from build123d import *

# Parameters (mm, degrees)
F0_W     = 36
F0_H     = 36
F1_DEPTH = 36
F2_W     = 21
F2_H     = 21
F3_DEPTH = 60
F4_R     = 2.5
F5_DEPTH = 25
F6_R     = 2.5
F7_DEPTH = 20
F8_R     = 4.25
F9_DEPTH = 5.5


with BuildPart() as f1:
    # F0 (on Front) → F1 (new body)
    with BuildSketch(Plane.XZ):
        with Locations((18, 18)):
            Rectangle(F0_W, F0_H)
    extrude(amount=F1_DEPTH)

    # F2 (on face) → F3 (cut)
    with BuildSketch(Plane.YZ.offset(36)):
        with Locations((-18, 18)):
            Rectangle(F2_W, F2_H)
    extrude(amount=-F3_DEPTH, mode=Mode.SUBTRACT)

    # F4 (on face) → F5 (cut)
    with BuildSketch(Plane.XY.offset(36)):
        with Locations((18, -18)):
            Circle(F4_R)
    extrude(amount=-F5_DEPTH, mode=Mode.SUBTRACT)

    # F6 (on face) → F7 (cut)
    with BuildSketch(Plane.XZ.offset(36)):
        with Locations((18, 18)):
            Circle(F6_R)
    extrude(amount=-F7_DEPTH, mode=Mode.SUBTRACT)

    # F8 (on face) → F9 (cut)
    with BuildSketch(Plane.XZ.offset(36)):
        with Locations((18, 18)):
            Circle(F8_R)
    extrude(amount=-F9_DEPTH, mode=Mode.SUBTRACT)


solid = f1.part
Can you work these out from the model? Positions are in its coordinate system, mm. A direction names the side the tool comes from. Give positions to 0.01 mm unless a question says otherwise; leave off trailing zeros. Loops run counter-clockwise (first coordinate to the right, second up) from the corner with the lowest first, then second, coordinate; pieces in that order, holes last. Notation, with made-up numbers: (-14.75, -15.5) -> (12.25, -15.5) arc R21 ccw to (12.25, -8.5) -> close; hole circle Ø11 at (28, 62.25). An arc over 180 degrees is marked (long way). Use one line per item in the form item = value.
1) If we section it at B-B (y = -23): Please give me the cut outline in (x, z), plus the area to 3 significant figures.
Answers:
outline = (0, 0) -> (36, 0) -> (36, 7.5) -> (0, 7.5) -> close; (0, 28.5) -> (36, 28.5) -> (36, 36) -> (0, 36) -> close
area = 540 mm²
2) I need wall thicknesses on line 1 along Z through (x, y) = (18, -29); line 2 along Z through (x, y) = (18, -11.5); line 3 along Y through (x, z) = (18, 32). Which ranges of each line are inside material? Lowest first, please.
Answers:
line_1 = 0 to 15.5, 20.5 to 36
line_2 = 0 to 7.5, 28.5 to 36
line_3 = -36 to -20.5, -15.5 to 0
3) If we section it at C-C (x = 18): Please give me the cut outline in (y, z), plus the area to 3 significant figures.
Answers:
outline = (-36, 0) -> (0, 0) -> (0, 36) -> (-15.5, 36) -> (-15.5, 28.5) -> (-7.5, 28.5) -> (-7.5, 7.5) -> (-28.5, 7.5) -> (-28.5, 15.5) -> (-30.5, 15.5) -> (-30.5, 13.75) -> (-36, 13.75) -> close; (-36, 22.25) -> (-30.5, 22.25) -> (-30.5, 20.5) -> (-28.5, 20.5) -> (-28.5, 28.5) -> (-20.5, 28.5) -> (-20.5, 36) -> (-36, 36) -> close
area = 761 mm²
4) For faces 1 (the face through (15.5, -17.9, 32.3)), 2 (the face through (14, -28.5, 18)), 3 (the face through (16.16, -29.51, 19.69)), which set-ups out of +Z, -Z, +X, -X, +Y, -Y let a thin tool reach every point of the face, with its end or its side?
Answers:
face_1 = +Z
face_2 = +X, -X
face_3 = -Y
5) If we section it at A-A (z = 20): Please give me the cut outline in (x, y), plus the area to 3 significant figures.
Answers:
outline = (0, -36) -> (14.25, -36) -> (14.25, -30.5) -> (16.5, -30.5) -> (16.5, -28.5) -> (0, -28.5) -> close; (0, -7.5) -> (36, -7.5) -> (36, 0) -> (0, 0) -> close; (19.5, -30.5) -> (21.75, -30.5) -> (21.75, -36) -> (36, -36) -> (36, -28.5) -> (19.5, -28.5) -> close
area = 493 mm²
6) If we section it at D-D (z = 24): Please give me the cut outline in (x, y), plus the area to 3 significant figures.
Answers:
outline = (0, -36) -> (36, -36) -> (36, -28.5) -> (0, -28.5) -> close; (0, -7.5) -> (36, -7.5) -> (36, 0) -> (0, 0) -> close
area = 540 mm²
7) Will these pins go through, and if not, where does the flat tip stop? pin 1 (7 mm diameter, centred on x = 18.5, z = 18.5, fed in from -Y); pin 2 (4 mm diameter, centred on x = 18, y = -18, fed in from +Z).
Answers:
pin_1 = -30.5
pin_2 = 7.5
8) We'd pull the mould along Z, two halves only. Please class faces 4 (the face through (14, -36, 22)), 5 (the face through (20, -30.5, 16)), 6 (the face through (17.08, -33.29, 13.85)), 7 (the face through (18, -18, 0)): released by +Z, released by -Z, zero draft, split by the parting line, or undercut.
Answers:
face_4 = zero draft
face_5 = undercut
face_6 = undercut
face_7 = released by -Z
